from build123d import *

# Parameters (mm, degrees)
SKETCH1_W               = 50.8
SKETCH1_H               = 25.4
BOSS_EXTRUDE1_DEPTH     = 254
SKETCH2_R               = 3.175
CUT_EXTRUDE1_DEPTH      = 25.4
FILLET2_R               = 25.4
FILLET1_R               = 2.54
CUT_EXTRUDE2_DEPTH      = 261.272549455
CUT_EXTRUDE2_DEPTH_BACK = 261.272549455
SKETCH3_R               = 3.175


with BuildPart() as part:
    # Sketch1 → Boss-Extrude1 (new body)
    with BuildSketch(Plane.XY):
        with Locations((-25.4, 12.7)):
            Rectangle(SKETCH1_W, SKETCH1_H)
    extrude(amount=BOSS_EXTRUDE1_DEPTH)

    # Sketch2 → Cut-Extrude1 (cut)
    with BuildSketch(Plane(origin=(0, 0, 0), x_dir=(-1, 0, 0), z_dir=(0, 0, -1))):
        with Locations((25.4, 12.7)):
            Circle(SKETCH2_R)
    extrude(amount=-CUT_EXTRUDE1_DEPTH, mode=Mode.SUBTRACT)

    # Fillet2
    fillet2_edges = [part.edges().sort_by_distance(p)[0] for p in [
        (0, 12.7, 254),
        (-50.8, 12.7, 254),
    ]]
    fillet(fillet2_edges, radius=FILLET2_R - 0.0001)  # a hair under: the kernel refuses the full size

    # Fillet1
    fillet1_edges = [part.edges().sort_by_distance(p)[0] for p in [
        (-50.8, 25.4, 114.30005),
        (0, 25.4, 114.30005),
        (-43.360541531, 25.4, 246.560541531),
        (-7.439458469, 25.4, 246.560541531),
        (0, 0, 114.30005),
        (-50.8, 0, 114.30005),
        (-43.360541531, 0, 246.560541531),
        (-7.439458469, 0, 246.560541531),
    ]]
    fillet(fillet1_edges, radius=FILLET1_R)

    # Sketch3 → Cut-Extrude2 (cut, two sides: drawn at the far end of the back side and taken through both)
    with BuildSketch(Plane(origin=(0, 25.4, 0), x_dir=(1, 0, 0), z_dir=(0, 1, 0)).offset(-CUT_EXTRUDE2_DEPTH_BACK)):
        with Locations(Location((-25.4, -228.6, 0), (0, 0, 180))):
            Circle(SKETCH3_R)
    extrude(amount=CUT_EXTRUDE2_DEPTH + CUT_EXTRUDE2_DEPTH_BACK, mode=Mode.SUBTRACT)


solid = part.part
CAD build for the part. Positions are in the model's coordinates, mm. Round coordinates to 2 decimals unless told otherwise and drop trailing zeros. Write each question's results on one line, items separated by ' | '.
1. Wall check: line 1 along Y through (x, z) = (-25.4, 18) (3 decimals); line 2 along Y through (x, z) = (-25, 7); line 3 along X through (y, z) = (15, 228.6) (3 decimals). Give the ranges that are in metal, low to high. Write a range as [from, to].
Findings below:
line 1: y = [0, 9.525], [15.875, 25.4] | line 2: y = [0, 9.55], [15.85, 25.4] | line 3: x = [-50.8, -28.575], [-22.225, 0]
2. Pull direction X, two halves, no side cores. Call faces 1 (the face through (-43.56, 12.84, 246.36)), 2 (the face through (-26, 0, 124)), 3 (the face through (-25, 13, 25.4)), 4 (the face through (-28.33, 11.48, 12.52)): pulls with the +X half, pulls with the -X half, needs draft (parallel to the pull), parting line crosses it, or undercut.
Findings below:
face 1: pulls with the -X half | face 2: needs draft | face 3: undercut | face 4: undercut
3. Flat gauge pin, fed straight in: P1, Ø5, axis at x = -43, y = 19.5, coming from the +Z side. Where does the tip first touch, or does it go through?
Findings below:
P1: stops at z = 249.02
